Part model, mm, in its own coordinate system. A direction names the side the tool comes from. Coordinates: 2 decimals unless noted, no trailing zeros. Loops run counter-clockwise (first coordinate to the right, second up) from the corner with the lowest first, then second, coordinate; pieces in that order, holes last. Notation, with made-up numbers: (-5, -15.75) -> (29, -15.75) arc R37 ccw to (29, 22.25) -> close; hole circle Ø4 at (16, 23). An arc over 180 degrees is marked (long way). Use one line per item in the form item = value. Start each with the question number.
(1) Drill centre lines: L1, parallel to Y at x = 27.5, z = 29; L2, parallel to Z at x = 43.5, y = 20.5; L3, parallel to X at y = 30, z = 6. Where is each one in solid material? Low to high. Write a range as [from, to].
(2) Band-saw the part on C-C on z = 2. Give the cut face in (x, y) (1 decimal).
(3) Pin check, flat tips, straight feed: P1, Ø10.5, axis at x = 28.5, y = 55.5, coming from the +Z side; P2, Ø5, axis at y = 58, z = -4.5, coming from the +X side; P3, Ø0.9, axis at x = 16, z = 1.5, coming from the +Y side. Stop position of each tip, or through.
(4) Band-saw the part on A-A on y = 13.5. Give the cut face in (x, z).
(5) Mould opens along X. For faces 1 (the flat face through (25, 62.611, -5)), 2 (the flat face through (40.513, 24, 17)), 3 (the cylindrical face through (42.3, 45.37, 1.55)) say: +X half, -X half, draft (parallel to the pull), parting line (faces both ways), or undercut.
(6) Band-saw the part on B-B on x = 10.5. Give the cut face in (y, z).
(7) 3-axis set-ups, long thin cutter, end or side, ignore diameter. For faces 4 (the flat face through (25, 56, 0)), 5 (the flat face through (24, 8.128, 17)), 6 (the flat face through (6.3, 8.4, 0)), 7 (the flat face through (37.148, 54, -5)), 8 (the flat face through (12.383, 54, -5)): which of +Z, -Z, +X, -X, +Y, -Y reach the whole face in a straight line?
(8) Band-saw the part on D-D on y = 57. Give the cut face in (x, z), then the cut area to 3 significant figures.
```python
from build123d import *

# Parameters (mm, degrees)
SKETCH1_W           = 49.53
SKETCH1_H           = 49.53
BOSS_EXTRUDE1_DEPTH = 3.048
SKETCH2_R           = 24.4475
BOSS_EXTRUDE2_DEPTH = 9.779
CUT_EXTRUDE1_START  = -9.779
SKETCH3_R           = 2.2225
CUT_EXTRUDE1_DEPTH  = 9.779
SKETCH4_W           = 31.75
SKETCH4_H           = 33.02
BOSS_EXTRUDE3_DEPTH = 27.94


with BuildPart() as part:
    # Sketch1 → Boss-Extrude1 (new body)
    with BuildSketch(Plane.XY):
        with Locations((24.765, 24.765)):
            Rectangle(SKETCH1_W, SKETCH1_H)
    extrude(amount=BOSS_EXTRUDE1_DEPTH)

    # Sketch2 → Boss-Extrude2 (add)
    with BuildSketch(Plane(origin=(0, 0, 0), x_dir=(-1, 0, 0), z_dir=(0, 0, -1))):
        Polygon((-37.1475, 49.53), (-24.765, 49.53), (-12.3825, 49.53), (-12.3825, 62.611), (-37.1475, 62.611), align=None)
        with BuildLine():
            Line((-12.3825, 49.53), (-24.765, 49.53))
            Line((-24.765, 49.53), (-37.1475, 49.53))
            Line((-37.1475, 49.53), (-37.1475, 45.844704694))
            ThreePointArc((-37.1475, 45.844704694), (-24.765, 49.2125), (-12.3825, 45.844704694))
            Line((-12.3825, 45.844704694), (-12.3825, 49.53))
        make_face()
        with Locations((-24.765, 24.765)):
            Circle(SKETCH2_R)
    extrude(amount=BOSS_EXTRUDE2_DEPTH)

    # Sketch3 → Cut-Extrude1 (cut)
    with BuildSketch(Plane(origin=(0, 0, 0), x_dir=(-1, 0, 0), z_dir=(0, 0, -1)).offset(CUT_EXTRUDE1_START)):
        with BuildLine():
            ThreePointArc((-41.449545605, 6.895859165), (-42.051993033, 7.478006967), (-42.634140835, 8.080454395))
            ThreePointArc((-42.634140835, 8.080454395), (-44.726461046, 7.884299394), (-45.72, 6.0325))
            Line((-45.72, 6.0325), (-43.4975, 6.0325))
            Line((-43.4975, 6.0325), (-43.4975, 3.81))
            ThreePointArc((-43.4975, 3.81), (-41.925955179, 4.460955179), (-41.275, 6.0325))
            ThreePointArc((-41.275, 6.0325), (-41.319073401, 6.472913219), (-41.449545605, 6.895859165))
        make_face()
        with BuildLine():
            Line((-43.4975, 6.0325), (-45.72, 6.0325))
            ThreePointArc((-45.72, 6.0325), (-45.069044821, 4.460955179), (-43.4975, 3.81))
            Line((-43.4975, 3.81), (-43.4975, 6.0325))
        make_face()
        with BuildLine():
            ThreePointArc((-6.859133168, 8.119874911), (-7.507381573, 7.448682191), (-8.180771601, 6.802716608))
            ThreePointArc((-8.180771601, 6.802716608), (-7.919638213, 4.762126071), (-6.096, 3.81))
            Line((-6.096, 3.81), (-6.096, 6.0325))
            Line((-6.096, 6.0325), (-3.8735, 6.0325))
            ThreePointArc((-3.8735, 6.0325), (-4.822531747, 7.853978756), (-6.859133168, 8.119874911))
        make_face()
        with BuildLine():
            Line((-6.096, 6.0325), (-6.096, 3.81))
            ThreePointArc((-6.096, 3.81), (-4.524455179, 4.460955179), (-3.8735, 6.0325))
            Line((-3.8735, 6.0325), (-6.096, 6.0325))
        make_face()
        with Locations((-6.0325, 43.434)):
            Circle(SKETCH3_R)
        with Locations((-43.4975, 43.4975)):
            Circle(SKETCH3_R)
    extrude(amount=CUT_EXTRUDE1_DEPTH, mode=Mode.SUBTRACT)

    # Sketch4 → Boss-Extrude3 (add)
    with BuildSketch(Plane.XY.offset(3.048)):
        with Locations((24.638, 24.638)):
            Rectangle(SKETCH4_W, SKETCH4_H)
    extrude(amount=BOSS_EXTRUDE3_DEPTH)


solid = part.part
```
A:
q1.L1 = [8.13, 41.15]
q1.L2 = [-9.78, 3.05]
q1.L3 = [8.76, 40.51]
q2.outline = (0, 0) -> (49.5, 0) -> (49.5, 49.5) -> (0, 49.5) -> close; hole circle Ø4.4 at (6, 43.4); hole (6.9, 8.1) arc R2.2 ccw (long way) to (8.2, 6.8) arc R24.4 cw to start; hole circle Ø4.4 at (43.5, 43.5); hole (41.4, 6.9) arc R2.2 ccw (long way) to (42.6, 8.1) arc R24.4 cw to start
q3.P1 = 0
q3.P2 = 37.15
q3.P3 = 49.53
q4.outline = (0, 0) -> (3.07, 0) -> (3.07, -9.78) -> (46.46, -9.78) -> (46.46, 0) -> (49.53, 0) -> (49.53, 3.05) -> (40.51, 3.05) -> (40.51, 30.99) -> (8.76, 30.99) -> (8.76, 3.05) -> (0, 3.05) -> close
q5.face_1 = draft
q5.face_2 = +X half
q5.face_3 = undercut
q6.outline = (0, 0) -> (4.91, 0) -> (4.91, -9.78) -> (44.62, -9.78) -> (44.62, 0) -> (49.53, 0) -> (49.53, 3.05) -> (41.15, 3.05) -> (41.15, 30.99) -> (8.13, 30.99) -> (8.13, 3.05) -> (0, 3.05) -> close
q7.face_4 = +Z, +X, -X, +Y
q7.face_5 = +Z, +X, -X, -Y
q7.face_6 = -Z
q7.face_7 = -Z, +X, +Y
q7.face_8 = -Z, -X, +Y
q8.outline = (12.38, -9.78) -> (37.15, -9.78) -> (37.15, 0) -> (12.38, 0) -> close
q8.area = 242 mm²
